Autodesk Fusion 360 part; units mm, degrees
sketch "Sketch1" plane through (0, 0, 0) normal (0, 1, 0) x (1, 0, 0)
  circle A0 centre (0, 0) radius 57.5
  line L0 (36, -36) -> (-36, -36) construction
  line L1 (-36, -36) -> (-36, 36) construction
  line L2 (-36, 36) -> (36, 36) construction
  line L3 (36, 36) -> (36, -36) construction
  line L4 (36, -36) -> (-36, 36) construction
  line L5 (-36, -36) -> (36, 36) construction
  circle A1 centre (0, 0) radius 43
  circle A2 centre (-36, 36) radius 2
  circle A3 centre (36, 36) radius 2
  circle A4 centre (36, -36) radius 2
  circle A5 centre (-36, -36) radius 2
  circle A6 centre (-36, -36) radius 2.875
  circle A7 centre (36, -36) radius 2.875
  circle A8 centre (36, 36) radius 2.875
  circle A9 centre (-36, 36) radius 2.875
  dimension "d1" = 115
  dimension "d2" = 72
  dimension "d3" = 72
  dimension "d4" = 86
  dimension "d5" = 4
  dimension "d6" = 4
  dimension "d7" = 4
  dimension "d8" = 4
  dimension "d9" = 5.75
  dimension "d10" = 5.75
  dimension "d11" = 5.75
  dimension "d12" = 5.75
extrude "Extrude1" add sketch "Sketch1" along normal blind 4 contours A0
extrude "Extrude3" add sketch "Sketch1" along normal blind 2 contours A1
sketch "Sketch2" plane through (0, 2, 0) normal (0, 1, 0) x (-1, 0, 0)
  circle A0 centre (0, 0) radius 43
  circle A1 centre (0, 0) radius 35 construction
  circle A2 centre (0, 0) radius 27.5 construction
  circle A3 centre (0, 0) radius 20 construction
  circle A4 centre (0, 0) radius 12.5 construction
  circle A5 centre (0, 0) radius 7.5 construction
  circle A6 centre (-0.2536, -34.9991) radius 3.5
  circle A7 centre (10.5741, -33.3645) radius 3.5
  circle A8 centre (20.3668, -28.4639) radius 3.5
  circle A9 centre (28.1658, -20.7771) radius 3.5
  circle A10 centre (33.2077, -11.0565) radius 3.5
  circle A11 centre (34.9991, -0.2536) radius 3.5
  circle A12 centre (33.3645, 10.5741) radius 3.5
  circle A13 centre (28.4639, 20.3668) radius 3.5
  circle A14 centre (20.7771, 28.1658) radius 3.5
  circle A15 centre (11.0565, 33.2077) radius 3.5
  circle A16 centre (0.2536, 34.9991) radius 3.5
  circle A17 centre (-10.5741, 33.3645) radius 3.5
  circle A18 centre (-20.3668, 28.4639) radius 3.5
  circle A19 centre (-28.1658, 20.7771) radius 3.5
  circle A20 centre (-33.2077, 11.0565) radius 3.5
  circle A21 centre (-34.9991, 0.2536) radius 3.5
  circle A22 centre (-33.3645, -10.5741) radius 3.5
  circle A23 centre (-28.4639, -20.3668) radius 3.5
  circle A24 centre (-20.7771, -28.1658) radius 3.5
  circle A25 centre (-11.0565, -33.2077) radius 3.5
  circle A26 centre (4.2963, -27.1623) radius 3.5
  circle A27 centre (12.4797, -24.5053) radius 3.5
  circle A28 centre (19.4414, -19.4495) radius 3.5
  circle A29 centre (24.5001, -12.4898) radius 3.5
  circle A30 centre (27.1605, -4.3076) radius 3.5
  circle A31 centre (27.1623, 4.2963) radius 3.5
  circle A32 centre (24.5053, 12.4797) radius 3.5
  circle A33 centre (19.4495, 19.4414) radius 3.5
  circle A34 centre (12.4898, 24.5001) radius 3.5
  circle A35 centre (4.3076, 27.1605) radius 3.5
  circle A36 centre (-4.2963, 27.1623) radius 3.5
  circle A37 centre (-12.4797, 24.5053) radius 3.5
  circle A38 centre (-19.4414, 19.4495) radius 3.5
  circle A39 centre (-24.5001, 12.4898) radius 3.5
  circle A40 centre (-27.1605, 4.3076) radius 3.5
  circle A41 centre (-27.1623, -4.2963) radius 3.5
  circle A42 centre (-24.5053, -12.4797) radius 3.5
  circle A43 centre (-19.4495, -19.4414) radius 3.5
  circle A44 centre (-12.4898, -24.5001) radius 3.5
  circle A45 centre (-4.3076, -27.1605) radius 3.5
  circle A46 centre (0.1335, -19.9996) radius 3.5
  circle A47 centre (11.8634, -16.1015) radius 3.5
  circle A48 centre (19.0619, -6.0533) radius 3.5
  circle A49 centre (18.9795, 6.3071) radius 3.5
  circle A50 centre (11.6475, 16.2584) radius 3.5
  circle A51 centre (-0.1335, 19.9996) radius 3.5
  circle A52 centre (-11.8634, 16.1015) radius 3.5
  circle A53 centre (-19.0619, 6.0533) radius 3.5
  circle A54 centre (-18.9795, -6.3071) radius 3.5
  circle A55 centre (-11.6475, -16.2584) radius 3.5
  circle A56 centre (4.3124, -11.7326) radius 3.5
  circle A57 centre (10.3851, -6.957) radius 3.5
  circle A58 centre (12.4909, 0.4758) radius 3.5
  circle A59 centre (9.8257, 7.7269) radius 3.5
  circle A60 centre (3.4074, 12.0266) radius 3.5
  circle A61 centre (-4.3124, 11.7326) radius 3.5
  circle A62 centre (-10.3851, 6.957) radius 3.5
  circle A63 centre (-12.4909, -0.4758) radius 3.5
  circle A64 centre (-9.8257, -7.7269) radius 3.5
  circle A65 centre (-3.4074, -12.0266) radius 3.5
  circle A66 centre (-0.0342, -5.0724) radius 2.5
  circle A67 centre (4.8135, -1.6) radius 2.5
  circle A68 centre (3.0092, 4.0835) radius 2.5
  circle A69 centre (-2.9538, 4.1238) radius 2.5
  circle A70 centre (-4.8347, -1.5349) radius 2.5
  dimension "d19" = 70
  dimension "d20" = 55
  dimension "d21" = 40
  dimension "d22" = 25
  dimension "d23" = 15
  dimension "d24" = 7
  dimension "d28" = 360
  dimension "d29" = 7
  dimension "d31" = 360
  dimension "d32" = 7
  dimension "d34" = 360
  dimension "d35" = 7
  dimension "d43" = 360
  dimension "d45" = 5
  dimension "d47" = 360
extrude "Extrude4" cut sketch "Sketch2" against normal up to surface (2 mm away) contours A6
extrude "Extrude5" cut sketch "Sketch2" against normal up to surface (2 mm away) contours A7 | A8 | A9 | A10 | A11 | A12 | A13 | A14 | A15 | A16 | A17 | A18 | A19 | A20 | A21 | A22 | A23 | A24 | A25 | A26 | A27 | A28 | A29 | A30 | A31 | A32 | A33 | A34 | A35 | A36 | A37 | A38 | A39 | A40 | A41 | A42 | A43 | A44 | A45 | A46 | A47 | A48 | A49 | A50 | A51 | A52 | A53 | A54 | A55 | A56 | A57 | A58 | A59 | A60 | A61 | A62 | A63 | A64 | A65 | A66 | A67 | A68 | A69 | A70
extrude "Extrude6" add sketch "Sketch1" against normal blind 2 from surface at 4 contours A6 | A7 | A8 | A9
chamfer "Chamfer1" distance 3 angle 45 1 edges at (-53.6088, 0, 20.7929)
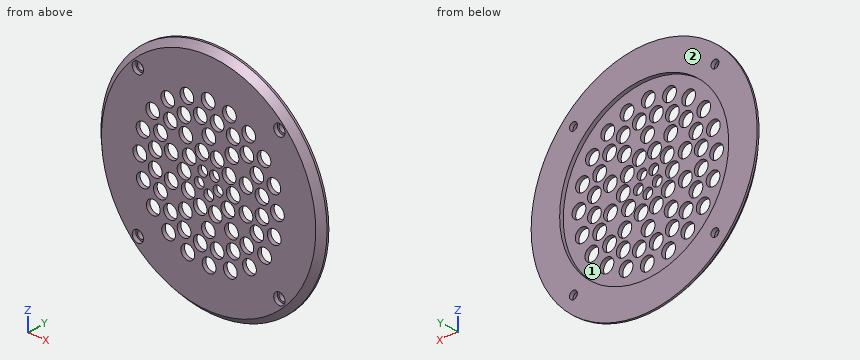
Verification items for the finished model (mm, model axes). Face numbers are marked on the shaded views. Coordinates: 2 decimals unless noted, no trailing zeros. One line per question, with ' | ' between items. Start each with the question number.
1. Draft check along X on the marked faces 1 and 2. Enter one of: released by +X, released by -X, zero draft, split by the parting line, or undercut.
2. Gauge pin test, flat ends, axial feed: P1, Ø5, axis at x = 2, z = 27, coming from the +Y side; P2, Ø5.5, axis at x = 10.57, z = 33.36, coming from the -Y side (3 decimals); P3, Ø12, axis at x = 45.5, z = -40, coming from the -Y side. Record the tip position at first contact, or that the pin passes through.
3. Material ranges on line 1 along X through (y, z) = (1.5, -36) (3 decimals); line 2 along X through (y, z) = (3.1, -1.5); line 3 along Z through (x, y) = (23, 0.3), recorded low to high.
Computed values:
1) face 1: undercut | face 2: zero draft
2) P1: y = 2 | P2: through | P3: y = 0.08
3) line 1: -42.895 to -38.875, -33.125 to -12.877, -8.271 to -3.1, 3.607 to 8.946, 13.167 to 33.125, 38.875 to 42.895 | line 2: -57.48 to -42.97, 42.97 to 57.48 | line 3: -49.74 to -30.87, -25.46 to -15.64, -9.32 to 9.33, 15.65 to 26.16, 30.77 to 49.74
